Geometry: final body of the model. Coordinates: model frame, mm. Coordinates: 2 decimals unless noted, no trailing zeros. Write each loop counter-clockwise with the first axis right and the second up, starting at its lowest first coordinate (ties: lowest second). Pieces come first, ordered by that corner, then holes. Notation, with made-up numbers: (16.5, 7.25) -> (26.5, 7.25) arc R26 cw to (26.5, 24.25) -> close; hole circle Ø4 at (18, 39.5). An arc over 180 degrees is marked (long way). Answer as a JSON object with one key per item and string values. Group by question number.
```python
from build123d import *

# Parameters (mm, degrees)
F1_DEPTH = 12.5


with BuildPart() as f1:
    # F0 (on Front) → F1 (new body, symmetric)
    with BuildSketch(Plane.XZ):
        Polygon((-205.444881, -174.193871), (-207.534229, -699.193871), (-207.534229, -724.193871), (-182.534427, -724.293363), (217.465573, -724.293363), (217.465573, -999.293363), (242.465355, -999.39783), (242.465355, -699.39783), (244.554703, -199.39783), (244.554722, -174.393082), (247.337235, 523.189536), (247.439954, 547.847293), (248.814853, 848.764804), (248.732482, 873.779536), (249.529363, 1074.015458), (249.529363, 1099.015458), (-175.370947, 1100.706637), (-200.370749, 1100.806129), (-201.266184, 875.806129), (-202.55959, 550.806129), align=None)
        Polygon((-182.534427, -699.293363), (-180.445079, -199.293363), (219.554921, -199.293363), (217.465573, -699.293363), align=None, mode=Mode.SUBTRACT)
        Polygon((219.554921, -174.293363), (-180.445079, -174.293363), (-177.662566, 524.88114), (222.337434, 523.289255), align=None, mode=Mode.SUBTRACT)
        Polygon((222.440212, 547.96088), (-177.559788, 550.706637), (-176.36681, 850.471637), (223.815114, 848.879028), align=None, mode=Mode.SUBTRACT)
        Polygon((223.73268, 873.879028), (-176.266382, 875.706637), (-175.470439, 1075.706835), (224.529561, 1074.11495), align=None, mode=Mode.SUBTRACT)
    extrude(amount=F1_DEPTH, both=True)


solid = f1.part
```
Item 1: Section A-A on x = -68. Output: boundary loops of the cut face in (y, z), then the cut area to 3 significant figures.
Item 2: Section B-B on z = -66. Output: boundary loops of the cut face in (x, y), then the cut area to 3 significant figures.
Item 3: Ray query, L1, parallel to Z at x = 216, y = 9.75; L2, parallel to Z at x = -160, y = 1; L3, parallel to X at y = -4.5, z = 814.5. Return the intervals inside material, ascending. Write a range as [from, to].
Item 4: Section C-C on y = -5.75. Give the number of separate pieces and of enclosed holes in the cut face, then the cut area to 3 significant figures.
Item 5: Section D-D on z = 675. Output: boundary loops of the cut face in (x, y).
Item 6: Contact query for flat-ended pins moving along their axis: pin 1 (12 mm diameter, centred on y = 0, z = 209.5, fed in from +X); pin 2 (8 mm diameter, centred on y = 1.5, z = 657, fed in from -X); pin 3 (6 mm diameter, centred on x = 188.5, y = 1.5, fed in from +Z). Output: stop coordinate, or through.
Answer sheet:
{
 "1": {"outline": "(-12.5, -724.29) -> (12.5, -724.29) -> (12.5, -699.29) -> (-12.5, -699.29) -> close; (-12.5, -199.29) -> (12.5, -199.29) -> (12.5, -174.29) -> (-12.5, -174.29) -> close; (-12.5, 524.44) -> (12.5, 524.44) -> (12.5, 549.95) -> (-12.5, 549.95) -> close; (-12.5, 850.04) -> (12.5, 850.04) -> (12.5, 875.21) -> (-12.5, 875.21) -> close; (-12.5, 1075.28) -> (12.5, 1075.28) -> (12.5, 1100.28) -> (-12.5, 1100.28) -> close", "area": "3,140 mm^2"},
 "2": {"outline": "(-205.01, -12.5) -> (-180.01, -12.5) -> (-180.01, 12.5) -> (-205.01, 12.5) -> close; (219.99, -12.5) -> (244.99, -12.5) -> (244.99, 12.5) -> (219.99, 12.5) -> close", "area": "1,250 mm^2"},
 "3": {"L1": "z = [-724.29, -699.29], [-199.29, -174.29], [523.31, 548.01], [848.91, 873.91], [1074.15, 1099.15]", "L2": "z = [-724.29, -699.29], [-199.29, -174.29], [524.81, 550.59], [850.41, 875.63], [1075.65, 1100.65]", "L3": "x = [-201.51, -176.51], [223.66, 248.66]"},
 "4": {"separate pieces": "1", "enclosed holes": "4", "area": "148,000 mm^2"},
 "5": {"outline": "(-202.07, -12.5) -> (-177.07, -12.5) -> (-177.07, 12.5) -> (-202.07, 12.5) -> close; (223.02, -12.5) -> (248.02, -12.5) -> (248.02, 12.5) -> (223.02, 12.5) -> close"},
 "6": {"pin 1": "stops at x = 246.11", "pin 2": "stops at x = -202.15", "pin 3": "stops at z = 1099.27"}
}
